Here's how the part is built. I have some questions about the finished solid (model axes, mm). Round coordinates to 2 decimals unless told otherwise and drop trailing zeros. Loops run counter-clockwise (first coordinate to the right, second up) from the corner with the lowest first, then second, coordinate; pieces in that order, holes last. Notation, with made-up numbers: M 3.5,5 L 10.5,5 A9 ccw 10.5,16 Z; hole C 79.25,54 d1. An arc over 180 degrees is marked long. Answer as a JSON object with one key per item and string values.
from build123d import *

# Parameters (mm, degrees)
F0_W     = 105
F0_H     = 130
F1_DEPTH = 3
F3_D     = 4.4
F4_R     = 8


with BuildPart() as f1:
    # F0 (on Front) → F1 (new body)
    with BuildSketch(Plane.XZ):
        Rectangle(F0_W, F0_H)
    extrude(amount=F1_DEPTH)

    # F3 (through all)
    with Locations(Plane.XZ.offset(3)):
        with Locations((-14, 0), (14, 0)):
            Hole(F3_D / 2)

    # F4
    f4_edges = [f1.edges().sort_by_distance(p)[0] for p in [
        (52.5, -1.5, 65),
        (-52.5, -1.5, 65),
        (-52.5, -1.5, -65),
        (52.5, -1.5, -65),
    ]]
    fillet(f4_edges, radius=F4_R)


solid = f1.part
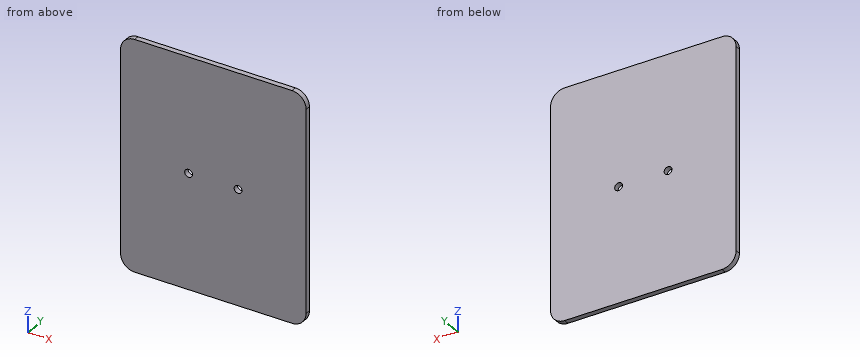
Item 1: I want a section at A-A on z = 0. List the corners of the cut face in (x, y) for me.
Solution:
{"outline": "M -52.5,-3 L -16.2,-3 L -16.2,0 L -52.5,0 Z; M -11.8,-3 L 11.8,-3 L 11.8,0 L -11.8,0 Z; M 16.2,-3 L 52.5,-3 L 52.5,0 L 16.2,0 Z"}
Item 2: If I drill on L1, parallel to Z at x = -14, y = -1.85; L2, parallel to Z at x = -45, y = -1.3; L3, parallel to Z at x = 16, y = -1.45, over which ranges is the centre line in solid material (lowest first)? Write a range as from..to.
Solution:
{"L1": "z = -65..-2.2, 2.2..65", "L2": "z = -64.98..64.98", "L3": "z = -65..-0.92, 0.92..65"}
Item 3: I want a section at B-B on x = 14. List the corners of the cut face in (y, z) for me.
Solution:
{"outline": "M -3,-65 L 0,-65 L 0,-2.2 L -3,-2.2 Z; M -3,2.2 L 0,2.2 L 0,65 L -3,65 Z"}
Item 4: For P1, Ø5, axis at x = 6, z = -24.5, coming from the +Y side; P2, Ø4, axis at x = -14, z = 0, coming from the +Y side, each with a flat end and sliding along its axis, tell me the tip position at first contact or that it passes through.
Solution:
{"P1": "stops at y = 0", "P2": "passes through"}
